Can you work these out from the drawing? Everything is in mm from the part's minimum corner. Round coordinates to 2 decimals unless told otherwise and drop trailing zeros. Write each loop counter-clockwise with the first axis right and the second up, starting at its lowest first coordinate (ties: lowest second). Pieces come first, ordered by that corner, then holes. Notation, with made-up numbers: (54.5, 22.5) - (97.5, 22.5) arc R8 cw to (97.5, 26.5) - close; hole circle Ø9 at (58, -12.5). An arc over 180 degrees is marked (long way). Write each question's results on one line, items separated by ' | '. Start each with the question number.
(1) Imagine slicing it at B-B on y = 0.8. Write out the boundary of the cut face in (x, z) (1 decimal).
(2) For P1, Ø5, axis at x = 32, z = 5.5, coming from the -Y side, with a flat end and sliding along its axis, tell me the tip position at first contact or that it passes through.
(3) Please list where these lines run through material, in increasing order: line 1 (X direction, y = 1.35, z = 12.7) (1 decimal); line 2 (X direction, y = 1.85, z = 13.5) (1 decimal); line 3 (Z direction, x = 11.5, y = 1) (1 decimal). Write a range as [from, to].
(4) Imagine slicing it at A-A on z = 12.7. Write out the boundary of the cut face in (x, y) (1 decimal).
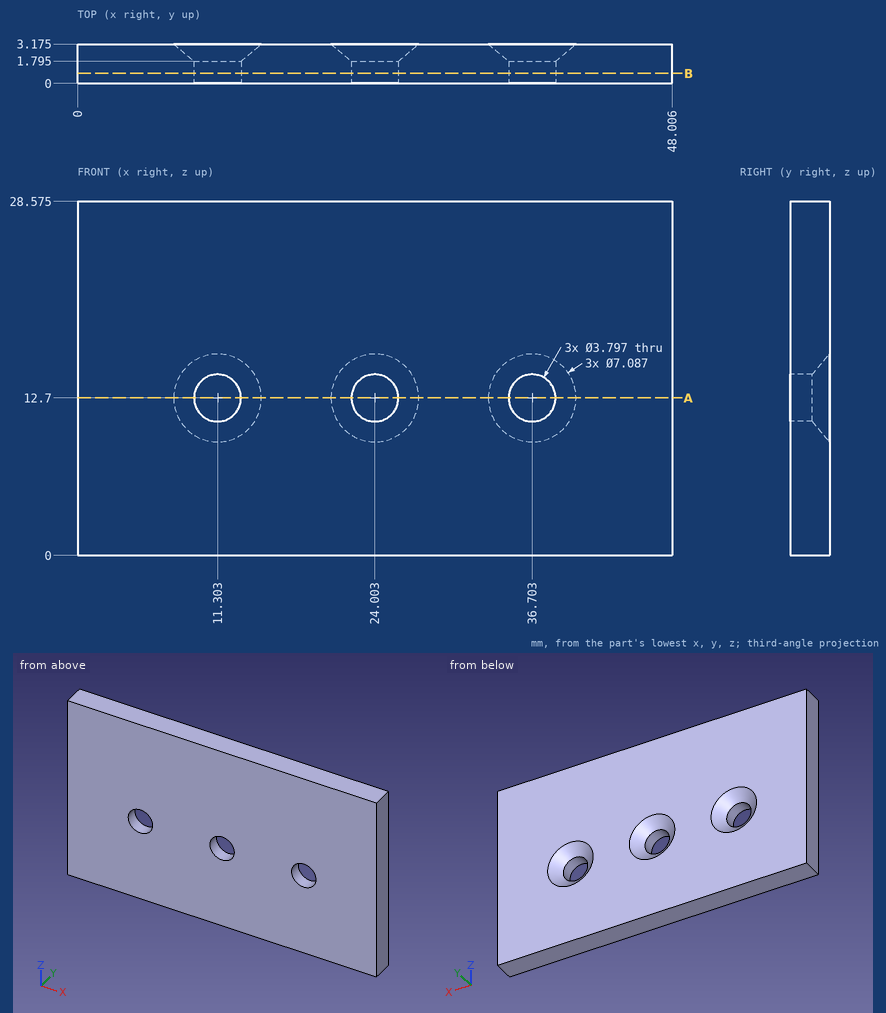
Response:
1) outline: (0, 0) - (48, 0) - (48, 28.6) - (0, 28.6) - close; hole circle Ø3.8 at (11.3, 12.7); hole circle Ø3.8 at (24, 12.7); hole circle Ø3.8 at (36.7, 12.7)
2) P1: y = 0
3) line 1: [0, 9.4], [13.2, 22.1], [25.9, 34.8], [38.6, 48] | line 2: [0, 9.5], [13.1, 22.2], [25.8, 34.9], [38.5, 48] | line 3: [0, 10.8], [14.6, 28.6]
4) outline: (0, 0) - (9.4, 0) - (9.4, 1.8) - (7.8, 3.2) - (0, 3.2) - close; (13.2, 0) - (22.1, 0) - (22.1, 1.8) - (20.5, 3.2) - (14.8, 3.2) - (13.2, 1.8) - close; (25.9, 0) - (34.8, 0) - (34.8, 1.8) - (33.2, 3.2) - (27.5, 3.2) - (25.9, 1.8) - close; (38.6, 0) - (48, 0) - (48, 3.2) - (40.2, 3.2) - (38.6, 1.8) - close
